from build123d import *

# Parameters (mm, degrees)
SKETCH_1_W          = 36
SKETCH_1_H          = 28
EXTRUDE_1_DEPTH     = 2
EXTRUDE_2_DEPTH     = 36
SKETCH_3_R          = 1.65
CUT_EXTRUDE_1_DEPTH = 4


with BuildPart() as part:
    # 草图1 → 凸台-拉伸1 (new body)
    with BuildSketch(Plane.XY):
        with Locations((18, 14)):
            Rectangle(SKETCH_1_W, SKETCH_1_H)
    extrude(amount=EXTRUDE_1_DEPTH)

    # 草图2 → 凸台-拉伸2 (add)
    with BuildSketch(Plane(origin=(36, 0, 0), x_dir=(0, 0, -1), z_dir=(1, 0, 0))):
        Polygon((-6.882121938, 32.882121938), (-2, 28), (0, 28), (-7.882121938, 35.882121938), (-32, 35.882121938), (-32, 32.882121938), align=None)
    extrude(amount=-EXTRUDE_2_DEPTH)

    # 草图3 → 切除-拉伸1 (cut)
    with BuildSketch(Plane.XY.offset(2)):
        with Locations((31, 23)):
            Circle(SKETCH_3_R)
        with Locations((6, 23)):
            Circle(SKETCH_3_R)
        with Locations((6, 8)):
            Circle(SKETCH_3_R)
        with Locations((31, 8)):
            Circle(SKETCH_3_R)
    extrude(amount=-CUT_EXTRUDE_1_DEPTH, mode=Mode.SUBTRACT)


solid = part.part
Here's how the part is built. I have some questions about the finished solid (model axes, mm). A direction names the side the tool comes from. Round coordinates to 2 decimals unless told otherwise and drop trailing zeros. Order: outer loops, then holes, each group sorted by start corner. A loop starts at its lowest first (then second) coordinate and runs counter-clockwise, first axis right, second up. Notation, with made-up numbers: (22.5, -4.5) -> (27.5, -4.5) arc R18 cw to (27.5, 15.5) -> close; hole circle Ø1 at (-18.75, 85.25). An arc over 180 degrees is marked (long way). Return JSON: item names as keys, results as strings.
Q1. I need wall thicknesses on line 1 along Y through (x, z) = (6, 1); line 2 along Y through (x, z) = (6, 0.55); line 3 along Y through (x, z) = (25, 23.5). Which ranges of each line are inside material? Lowest first, please. Write a range as from..to.
Filled sheet:
{"line 1": "y = 0..6.35, 9.65..21.35, 24.65..29", "line 2": "y = 0..6.35, 9.65..21.35, 24.65..28.55", "line 3": "y = 32.88..35.88"}
Q2. If we section it at C-C on x = 17: List the corners of the cut face in (y, z) for me.
Filled sheet:
{"outline": "(0, 0) -> (28, 0) -> (35.88, 7.88) -> (35.88, 32) -> (32.88, 32) -> (32.88, 6.88) -> (28, 2) -> (0, 2) -> close"}
Q3. If we section it at A-A on y = 23: List the corners of the cut face in (x, z) for me, plus the area to 3 significant figures.
Filled sheet:
{"outline": "(0, 0) -> (4.35, 0) -> (4.35, 2) -> (0, 2) -> close; (7.65, 0) -> (29.35, 0) -> (29.35, 2) -> (7.65, 2) -> close; (32.65, 0) -> (36, 0) -> (36, 2) -> (32.65, 2) -> close", "area": "58.8 mm^2"}
Q4. If we mould it in two halves opening along X, with no side actions, what happens to faces 1 (the flat face through (18, 14, 2)), 2 (the cylindrical face through (4.784, 9.115, 1.014))? For each: released by +X, released by -X, zero draft, split by the parting line, or undercut.
Filled sheet:
{"face 1": "zero draft", "face 2": "undercut"}
Q5. If we section it at D-D on z = 22: List the corners of the cut face in (x, y) for me, plus the area to 3 significant figures.
Filled sheet:
{"outline": "(0, 32.88) -> (36, 32.88) -> (36, 35.88) -> (0, 35.88) -> close", "area": "108 mm^2"}
Q6. For pin 1 Ø2 at (x, y) = (13.5, 29.5) entering from -Z; pin 2 Ø1 at (x, y) = (24.5, 30.5) entering from -Z; pin 3 Ø14 at (x, y) = (13, 7.5) entering from +Z, each with a flat end and sliding along its axis, tell me the tip position at first contact or that it passes through.
Filled sheet:
{"pin 1": "stops at z = 0.5", "pin 2": "stops at z = 2", "pin 3": "stops at z = 2"}
Q7. If we section it at B-B on x = 31: List the corners of the cut face in (y, z) for me, plus the area to 3 significant figures.
Filled sheet:
{"outline": "(0, 0) -> (6.35, 0) -> (6.35, 2) -> (0, 2) -> close; (9.65, 0) -> (21.35, 0) -> (21.35, 2) -> (9.65, 2) -> close; (24.65, 0) -> (28, 0) -> (35.88, 7.88) -> (35.88, 32) -> (32.88, 32) -> (32.88, 6.88) -> (28, 2) -> (24.65, 2) -> close", "area": "129 mm^2"}
Q8. Which directions (+Z, -Z, +X, -X, +Y, -Y) give clear straight access to the entire face, cutting with the end or side of a thin tool? Please do faces 3 (the cylindrical face through (29.35, 8.07, 1.01)), 4 (the flat face through (18, 32.882, 20)).
Filled sheet:
{"face 3": "+Z, -Z", "face 4": "+Z, +X, -X, -Y"}
